The listing builds one solid part. Answer for the finished solid, in the listing's coordinates (mm). Coordinates: 2 decimals unless noted, no trailing zeros. Loops run counter-clockwise (first coordinate to the right, second up) from the corner with the lowest first, then second, coordinate; pieces in that order, holes last. Notation, with made-up numbers: (39.25, 28) -> (51.25, 28) arc R27 cw to (51.25, 52) -> close; hole circle Ø2 at (-25, 71.25). An arc over 180 degrees is marked (long way). Answer in a Markdown table with one row per item.
```python
from build123d import *

# Parameters (mm, degrees)
SKETCH1_W           = 152.4
SKETCH1_H           = 88.9
SKETCH1_R           = 3.3782
SKETCH1_R_2         = 6.35
SKETCH1_R_3         = 22.225
BOSS_EXTRUDE1_DEPTH = 3.175
SKETCH2_R           = 3.3782
CUT_EXTRUDE1_DEPTH  = 4.175
SKETCH3_W           = 152.4
SKETCH3_H           = 25.4
CUT_EXTRUDE2_DEPTH  = 4.175
FILLET1_R           = 6.35


with BuildPart() as part:
    # Sketch1 → Boss-Extrude1 (new body)
    with BuildSketch(Plane.XY):
        Rectangle(SKETCH1_W, SKETCH1_H)
        with Locations((-28.575, 0)):
            Circle(SKETCH1_R, mode=Mode.SUBTRACT)
        with Locations((0, 28.575)):
            Circle(SKETCH1_R, mode=Mode.SUBTRACT)
        with Locations((28.575, 0)):
            Circle(SKETCH1_R, mode=Mode.SUBTRACT)
        with Locations((0, -28.575)):
            Circle(SKETCH1_R, mode=Mode.SUBTRACT)
        with Locations((-57.15, 0)):
            Circle(SKETCH1_R_2, mode=Mode.SUBTRACT)
        with Locations((57.15, 0)):
            Circle(SKETCH1_R_2, mode=Mode.SUBTRACT)
        Circle(SKETCH1_R_3, mode=Mode.SUBTRACT)
    extrude(amount=BOSS_EXTRUDE1_DEPTH)

    # Sketch2 → Cut-Extrude1 (cut, through all)
    with BuildSketch(Plane.XY.offset(3.175)):
        with BuildLine():
            Line((-28.575, -20.32), (-28.575, -44.45))
            Line((-28.575, -44.45), (28.575, -44.45))
            Line((28.575, -44.45), (28.575, -20.32))
            Line((28.575, -20.32), (22.225, -20.32))
            Line((22.225, -20.32), (9.002678768, -20.32))
            ThreePointArc((9.002678768, -20.32), (0, -22.225), (-9.002678768, -20.32))
            Line((-9.002678768, -20.32), (-22.225, -20.32))
            Line((-22.225, -20.32), (-28.575, -20.32))
        make_face()
        with Locations((0, -28.575)):
            Circle(SKETCH2_R, mode=Mode.SUBTRACT)
        with BuildLine():
            Line((-22.225, 0), (-22.225, -20.32))
            Line((-22.225, -20.32), (-9.002678768, -20.32))
            ThreePointArc((-9.002678768, -20.32), (-18.628407884, -12.121594148), (-22.225, 0))
        make_face()
        with BuildLine():
            Line((9.002678768, -20.32), (22.225, -20.32))
            Line((22.225, -20.32), (22.225, 0))
            ThreePointArc((22.225, 0), (18.628407884, -12.121594148), (9.002678768, -20.32))
        make_face()
        with BuildLine():
            ThreePointArc((-22.225, 0), (-18.628407884, -12.121594148), (-9.002678768, -20.32))
            Line((-9.002678768, -20.32), (9.002678768, -20.32))
            ThreePointArc((9.002678768, -20.32), (18.628407884, -12.121594148), (22.225, 0))
            Line((22.225, 0), (-22.225, 0))
        make_face()
        with BuildLine():
            Line((9.002678768, -20.32), (-9.002678768, -20.32))
            ThreePointArc((-9.002678768, -20.32), (0, -22.225), (9.002678768, -20.32))
        make_face()
    extrude(amount=-CUT_EXTRUDE1_DEPTH, mode=Mode.SUBTRACT)

    # Sketch3 → Cut-Extrude2 (cut, through all)
    with BuildSketch(Plane.XY.offset(3.175)):
        with Locations((0, -31.75)):
            Rectangle(SKETCH3_W, SKETCH3_H)
    extrude(amount=-CUT_EXTRUDE2_DEPTH, mode=Mode.SUBTRACT)

    # Fillet1
    fillet1_edges = [part.edges().sort_by_distance(p)[0] for p in [
        (-76.2, 44.45, 1.5875),
        (76.2, 44.45, 1.5875),
        (-76.2, -19.05, 1.5875),
        (76.2, -19.05, 1.5875),
    ]]
    fillet(fillet1_edges, radius=FILLET1_R)


solid = part.part
```
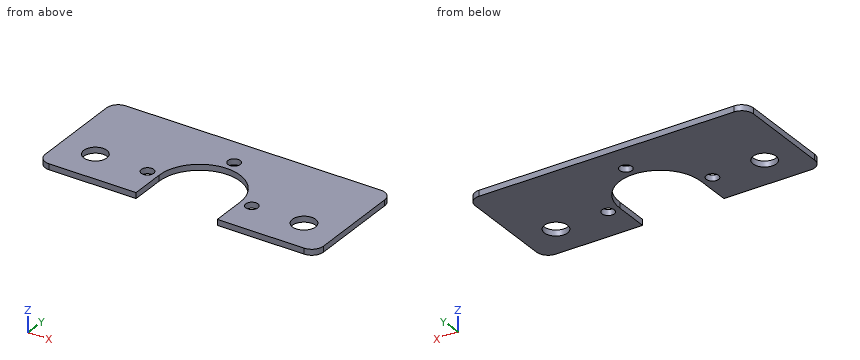
Item 1: Find the intervals of material crossed by probe 1 along Y at (x, z) = (0, 2.4) (3 decimals); probe 2 along X at (y, z) = (-13, 1.1) (3 decimals); probe 3 along X at (y, z) = (19, 0.2), in increasing order.
Findings below:
| item | result |
|---|---|
| probe 1 | y = 22.225 to 25.197, 31.953 to 44.45 |
| probe 2 | x = -76.193 to -22.225, 22.225 to 76.193 |
| probe 3 | x = -76.2 to -11.53, 11.53 to 76.2 |
Item 2: Flat-ended cylindrical pins translate along their axes: pin 1 Ø9 at (x, y) = (-28.575, 0) entering from -Z; pin 2 Ø6 at (x, y) = (28.575, 0) entering from -Z. Find the tip coordinate at first contact, or state that the pin passes through.
Findings below:
| item | result |
|---|---|
| pin 1 | stops at z = 0 |
| pin 2 | passes through |
Item 3: A cutting plane is placed at C-C, the plane z = 1.2. Determine the outline of the cut face in (x, y) (3 decimals), plus the area to 3 significant figures.
Findings below:
| item | result |
|---|---|
| outline | (-76.2, -12.7) arc R6.35 ccw to (-69.85, -19.05) -> (-22.225, -19.05) -> (-22.225, 0) arc R22.225 cw to (22.225, 0) -> (22.225, -19.05) -> (69.85, -19.05) arc R6.35 ccw to (76.2, -12.7) -> (76.2, 38.1) arc R6.35 ccw to (69.85, 44.45) -> (-69.85, 44.45) arc R6.35 ccw to (-76.2, 38.1) -> close; hole circle Ø12.7 at (-57.15, 0); hole circle Ø6.756 at (-28.575, 0); hole circle Ø6.756 at (0, 28.575); hole circle Ø6.756 at (28.575, 0); hole circle Ø12.7 at (57.15, 0) |
| area | 7,660 mm2 |
Item 4: A cutting plane is placed at B-B, the plane y = 12. Determine the outline of the cut face in (x, z) (3 decimals), plus the area to 3 significant figures.
Findings below:
| item | result |
|---|---|
| outline | (-76.2, 0) -> (-18.707, 0) -> (-18.707, 3.175) -> (-76.2, 3.175) -> close; (18.707, 0) -> (76.2, 0) -> (76.2, 3.175) -> (18.707, 3.175) -> close |
| area | 365 mm2 |
Item 5: A cutting plane is placed at A-A, the plane x = -57.15. Determine the outline of the cut face in (y, z) (3 decimals).
Findings below:
| item | result |
|---|---|
| outline | (-19.05, 0) -> (-6.35, 0) -> (-6.35, 3.175) -> (-19.05, 3.175) -> close; (6.35, 0) -> (44.45, 0) -> (44.45, 3.175) -> (6.35, 3.175) -> close |
